Model file for the job. Use its own axes, mm. Face numbers are marked on the shaded views. A direction names the side the tool comes from. Coordinates: 2 decimals unless noted, no trailing zeros. Write each loop counter-clockwise with the first axis right and the second up, starting at its lowest first coordinate (ties: lowest second). Pieces come first, ordered by that corner, then holes. Notation, with made-up numbers: M 18,24 L 77,24 A25 ccw 77,47 Z; hole C 77.25,42 d10. An arc over 180 degrees is marked long. One line per question, with ' | ' between items. Start each with the question number.
(1) Cut at A-A (x = -69.5). Write the cut outline in (y, z).
(2) Flat gauge pins, fed straight in: pin 1 Ø6 at (y, z) = (-10.5, 11.5) entering from +X; pin 2 Ø15 at (x, z) = (-10, 58) entering from +Y; pin 3 Ø24.5 at (x, y) = (31, -9.5) entering from +Z. Where does each tip first touch, or does it go through?
(3) Two-plate mould, pull along Z, no slides. Class the marked faces 1, 2 and 3: +Z half, -Z half, draft (parallel to the pull), parting line (faces both ways), or undercut.
(4) Wall check: probe 1 along Z at (x, y) = (45, -8); probe 2 along X at (y, z) = (2.5, 66); probe 3 along X at (y, z) = (-22, 6). Give the ranges that are in metal, low to high.
(5) Cut at B-B (z = 24.5). Write the cut outline in (x, y).
(6) Cut at C-C (x = 22). Write the cut outline in (y, z), plus the area to 3 significant figures.
(7) Tool access for the marked faces 4, 5 and 6: list every direction of +Z, -Z, +X, -X, +Y, -Y with a clear straight run to the whole face (end or side of a thin tool).
(8) Cut at D-D (z = 34.5). Write the cut outline in (x, y).
from build123d import *

# Parameters (mm, degrees)
Y_KSEKLIK_EKSTR_ZYON1_DEPTH = 75
IZIM3_W                     = 19
IZIM3_H                     = 64
Y_KSEKLIK_EKSTR_ZYON6_DEPTH = 77
RADYUS1_RADIUS              = 32
RADYUS1_LENGTH              = 19
RADYUS2_RADIUS              = 32
RADYUS2_LENGTH              = 19
KES_EKSTR_ZYON1_DEPTH       = 120.031428784
KES_EKSTR_ZYON1_DEPTH_BACK  = 120.031428784
IZIM4_R                     = 12.5
IZIM6_W                     = 21
IZIM6_H                     = 75
Y_KSEKLIK_EKSTR_ZYON7_DEPTH = 28
KES_EKSTR_ZYON3_REACH       = 111.469


with BuildPart() as part:
    # Çizim1 → Yükseklik-Ekstrüzyon1 (new body)
    with BuildSketch(Plane.XY):
        Polygon((-87.576185102, -10.168171558), (-87.576185102, -30.168171558), (-24.576185102, -30.168171558), (-24.576185102, 44.831828442), (-87.576185102, 44.831828442), (-87.576185102, 24.831828442), (-49.576185102, 24.831828442), (-49.576185102, -10.168171558), align=None)
    extrude(amount=Y_KSEKLIK_EKSTR_ZYON1_DEPTH)

    # Çizim3 → Yükseklik-Ekstrüzyon6 (add)
    with BuildSketch(Plane(origin=(-24.576185102, 0, 0), x_dir=(0, 0, -1), z_dir=(1, 0, 0))):
        with Locations((-57.5, 1.831828442)):
            Rectangle(IZIM3_W, IZIM3_H)
        with Locations((-17.5, 1.831828442)):
            Rectangle(IZIM3_W, IZIM3_H)
    extrude(amount=Y_KSEKLIK_EKSTR_ZYON6_DEPTH)

    # Radyus1: full round fillet: the end face becomes a half cylinder, R = half its width
    radyus1_face = Plane((52.423814898, 1.831828442, 57.5), x_dir=(0, 0, 1), z_dir=(1, 0, 0))  # on the end face: x along it, z out of the body
    radyus1_slab = radyus1_face.offset(-RADYUS1_RADIUS / 2) * Box(RADYUS1_LENGTH, 2 * RADYUS1_RADIUS, RADYUS1_RADIUS, mode=Mode.PRIVATE)  # the body's end, R deep
    radyus1_round = Plane((20.423814898, 1.831828442, 57.5), x_dir=(1, 0, 0), z_dir=(0, 0, 1)) * Cylinder(RADYUS1_RADIUS, RADYUS1_LENGTH, mode=Mode.PRIVATE)  # its axis R under the face
    add(radyus1_slab - radyus1_round, mode=Mode.SUBTRACT)

    # Radyus2: full round fillet: the end face becomes a half cylinder, R = half its width
    radyus2_face = Plane((52.423814898, 1.831828442, 17.5), x_dir=(0, 0, 1), z_dir=(1, 0, 0))  # on the end face: x along it, z out of the body
    radyus2_slab = radyus2_face.offset(-RADYUS2_RADIUS / 2) * Box(RADYUS2_LENGTH, 2 * RADYUS2_RADIUS, RADYUS2_RADIUS, mode=Mode.PRIVATE)  # the body's end, R deep
    radyus2_round = Plane((20.423814898, 1.831828442, 17.5), x_dir=(1, 0, 0), z_dir=(0, 0, 1)) * Cylinder(RADYUS2_RADIUS, RADYUS2_LENGTH, mode=Mode.PRIVATE)  # its axis R under the face
    add(radyus2_slab - radyus2_round, mode=Mode.SUBTRACT)

    # Çizim4 → Kes-Ekstrüzyon1 (cut, two sides: drawn at the far end of the back side and taken through both)
    with BuildSketch(Plane.XY.offset(67).offset(-KES_EKSTR_ZYON1_DEPTH_BACK)):
        with Locations(Location((20.423814898, 1.831828442, 0), (0, 0, 90))):
            Circle(IZIM4_R)
    extrude(amount=KES_EKSTR_ZYON1_DEPTH + KES_EKSTR_ZYON1_DEPTH_BACK, mode=Mode.SUBTRACT)

    # Çizim6 → Yükseklik-Ekstrüzyon7 (add)
    with BuildSketch(Plane(origin=(-24.576185102, 0, 0), x_dir=(0, 0, -1), z_dir=(1, 0, 0))):
        with Locations((-37.5, 7.331828442)):
            Rectangle(IZIM6_W, IZIM6_H)
    extrude(amount=Y_KSEKLIK_EKSTR_ZYON7_DEPTH)

    # Çizim7 → Kes-Ekstrüzyon3 (cut, up to next)
    with BuildSketch(Plane.XY.offset(48), mode=Mode.PRIVATE) as kes_ekstr_zyon3_sk1:
        Polygon((-24.576185102, 44.831828442), (3.423814898, 33.831828442), (3.423814898, 44.831828442), align=None)
    kes_ekstr_zyon3_tool1 = extrude(kes_ekstr_zyon3_sk1.sketch, amount=-KES_EKSTR_ZYON3_REACH, mode=Mode.PRIVATE) & part.part
    add(kes_ekstr_zyon3_tool1.solids().sort_by_distance((-5.909518, 41.165162, 48))[0], mode=Mode.SUBTRACT)


solid = part.part
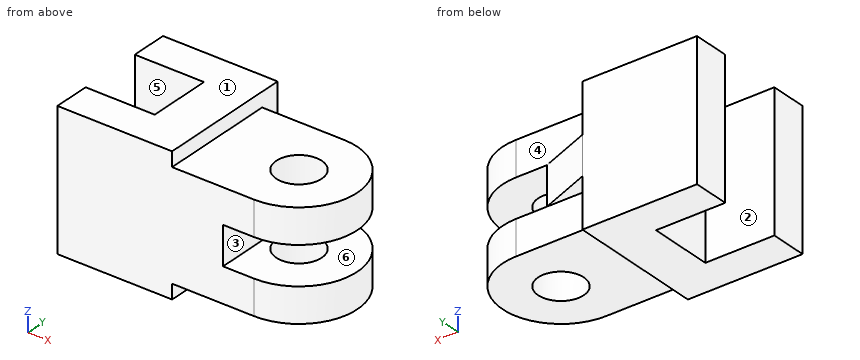
Filled in:
1) outline: M -30.17,0 L -10.17,0 L -10.17,75 L -30.17,75 Z; M 24.83,0 L 44.83,0 L 44.83,75 L 24.83,75 Z
2) pin 1: x = 51.03 | pin 2: y = 33.83 | pin 3: z = 67
3) face 1: +Z half | face 2: draft | face 3: undercut
4) probe 1: 8 to 27, 48 to 67 | probe 2: -49.58 to 7.94, 32.91 to 52.42 | probe 3: -87.58 to -24.58
5) outline: M -87.58,-30.17 L 20.42,-30.17 A32 ccw 20.42,33.83 L -24.58,33.83 L -24.58,44.83 L -87.58,44.83 L -87.58,24.83 L -49.58,24.83 L -49.58,-10.17 L -87.58,-10.17 Z; hole C 20.42,1.83 d25
6) outline: M -30.13,8 L -10.57,8 L -10.57,27 L -30.13,27 Z; M -30.13,48 L -10.57,48 L -10.57,67 L -30.13,67 Z; M 14.23,8 L 33.79,8 L 33.79,27 L 14.23,27 Z; M 14.23,48 L 33.79,48 L 33.79,67 L 14.23,67 Z | area: 1,490 mm²
7) face 4: +Z, +X, +Y | face 5: +Z, -Z, -X | face 6: +X, +Y, -Y
8) outline: M -87.58,-30.17 L 3.42,-30.17 L 3.42,33.83 L -24.58,44.83 L -87.58,44.83 L -87.58,24.83 L -49.58,24.83 L -49.58,-10.17 L -87.58,-10.17 Z
